Study the drawing (mm; zero at the part's minimum x, y, z) and answer. Coordinates: 2 decimals unless noted, no trailing zeros. Loops run counter-clockwise (first coordinate to the right, second up) from the corner with the lowest first, then second, coordinate; pieces in that order, holes last. Notation, with made-up numbers: (75, -36) -> (107, -36) arc R8 ccw to (107, -31) -> close; hole circle Ø2 at (52.5, 64). An arc over 180 degrees is marked (long way). Answer in a Markdown table with one row per item.
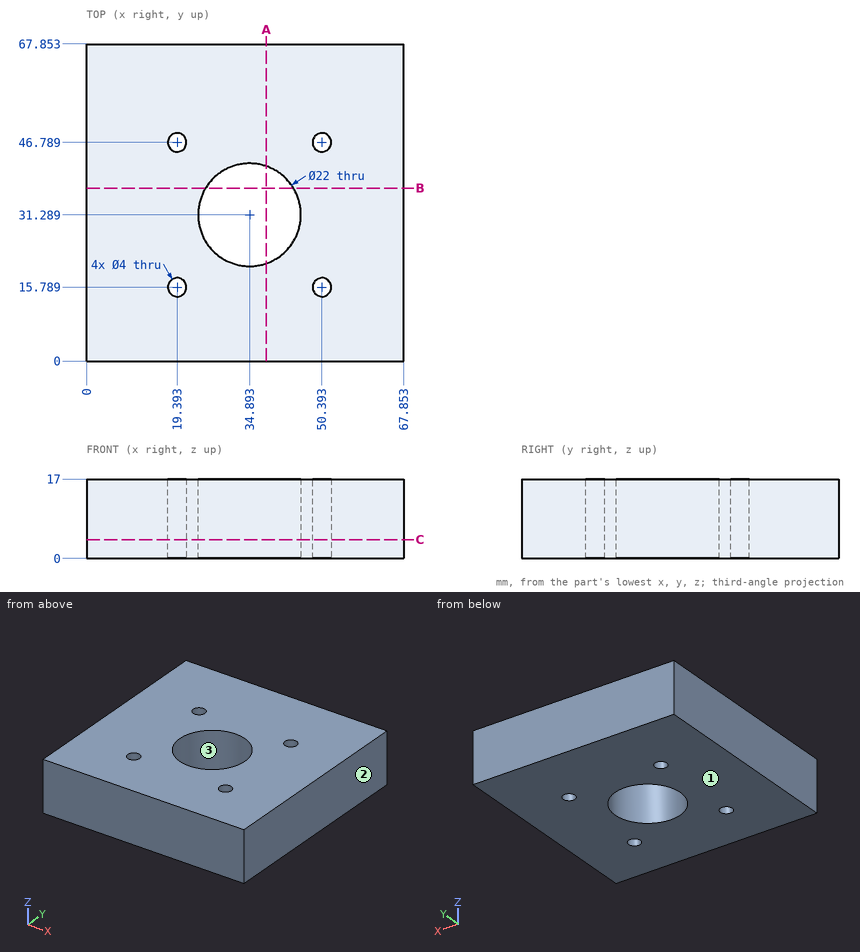
1. A cutting plane is placed at C-C on z = 4. Give the vertices of the cut face in (x, y).
A:
| item | result |
|---|---|
| outline | (0, 0) -> (67.85, 0) -> (67.85, 67.85) -> (0, 67.85) -> close; hole circle Ø4 at (19.39, 15.79); hole circle Ø4 at (19.39, 46.79); hole circle Ø22 at (34.89, 31.29); hole circle Ø4 at (50.39, 15.79); hole circle Ø4 at (50.39, 46.79) |
2. The mould has two halves that part along X. Classify the marked faces 1, 2 and 3: pulls with the +X half, pulls with the -X half, needs draft (parallel to the pull), parting line crosses it, or undercut.
A:
| item | result |
|---|---|
| face 1 | needs draft |
| face 2 | pulls with the +X half |
| face 3 | undercut |
3. Given pin 1 Ø3 at (x, y) = (19.39, 15.79) entering from -Z, flat-ended and moving along its own axis, determine where the tip first touches the part or whether it passes through.
A:
| item | result |
|---|---|
| pin 1 | passes through |
4. A cutting plane is placed at A-A on x = 38.5. Give the vertices of the cut face in (y, z).
A:
| item | result |
|---|---|
| outline | (0, 0) -> (20.9, 0) -> (20.9, 17) -> (0, 17) -> close; (41.68, 0) -> (67.85, 0) -> (67.85, 17) -> (41.68, 17) -> close |
5. Find the intervals of material crossed by probe 1 along Y at (x, z) = (50.5, 3.25); probe 2 along X at (y, z) = (47, 1); probe 3 along Y at (x, z) = (49.5, 15.75), in increasing order.
A:
| item | result |
|---|---|
| probe 1 | y = 0 to 13.79, 17.79 to 44.79, 48.79 to 67.85 |
| probe 2 | x = 0 to 17.4, 21.38 to 48.4, 52.38 to 67.85 |
| probe 3 | y = 0 to 14, 17.58 to 45, 48.58 to 67.85 |
6. A cutting plane is placed at B-B on y = 37. Give the vertices of the cut face in (x, z) (1 decimal).
A:
| item | result |
|---|---|
| outline | (0, 0) -> (25.5, 0) -> (25.5, 17) -> (0, 17) -> close; (44.3, 0) -> (67.9, 0) -> (67.9, 17) -> (44.3, 17) -> close |
